Here's how the part is built. I have some questions about the finished solid (model axes, mm). A direction names the side the tool comes from. Round coordinates to 2 decimals unless told otherwise and drop trailing zeros. Loops run counter-clockwise (first coordinate to the right, second up) from the corner with the lowest first, then second, coordinate; pieces in that order, holes last. Notation, with made-up numbers: M 73,84.25 L 78,84.25 A13 cw 78,104.25 Z; hole C 7.5,82 d11. An arc over 180 degrees is marked long. Write each question's results on one line, items separated by ' | '. Start each with the question number.
```python
from build123d import *

# Parameters (mm, degrees)
F0_R     = 0.762
F1_DEPTH = 7.9248
F2_R     = 1.524
F3_DEPTH = 32.005


with BuildPart() as f1:
    # F0 (on Top) → F1 (new body)
    with BuildSketch(Plane.XY):
        Polygon((32.004, 34.163), (32.004, 40.513), (12.319, 40.513), (12.319, 34.29), (5.08, 34.29), (0, 29.21), (0, 0), (6.985, -6.985), (13.589, -6.985), (13.589, -11.303), (16.764, -11.303), (16.764, -6.985), (20.32, -6.985), (20.32, 22.733), align=None)
        with Locations((22.098, 33.909)):
            Circle(F0_R, mode=Mode.SUBTRACT)
    extrude(amount=F1_DEPTH)

    # F2 (on Right) → F3 (cut, through all)
    with BuildSketch(Plane.YZ):
        with Locations((37.3888, 4.064)):
            Circle(F2_R)
        with BuildLine():
            Line((-11.303, 2.54), (-9.3472, 2.54))
            ThreePointArc((-9.3472, 2.54), (-7.8232, 4.064), (-9.3472, 5.588))
            Line((-9.3472, 5.588), (-11.303, 5.588))
            Line((-11.303, 5.588), (-11.303, 2.54))
        make_face()
    extrude(amount=F3_DEPTH, mode=Mode.SUBTRACT)


solid = f1.part
```
1. I need wall thicknesses on line 1 along X through (y, z) = (15.5, 3.75); line 2 along X through (y, z) = (-8, 5); line 3 along Y through (x, z) = (12.5, 6.75) (3 decimals). Which ranges of each line are inside material? Lowest first, please.
2. Which directions (+Z, -Z, +X, -X, +Y, -Y) give clear straight access to the entire face, cutting with the end or side of a thin tool? Please do faces 4 (the face through (15, -10, 5.588)), 5 (the face through (13.589, -8, 3)), 6 (the face through (12.319, 39, 3)).
3. I want a section at B-B on x = 22. List the corners of the cut face in (y, z) for me, plus the area to 3 significant figures.
4. For pin 1 (4 mm diameter, centred on x = 19, z = 4, fed in from -Y) (3 decimals); pin 2 (1.2 mm diameter, centred on x = 22.098, y = 33.909, fed in from -Z); pin 3 (3 mm diameter, centred on x = 18, z = 4, fed in from -Y); pin 4 (4 mm diameter, centred on x = 7, z = 4.5, fed in from +Y), each with a flat end and sliding along its axis, tell me the tip position at first contact or that it passes through.
5. I want a section at D-D on y = 22. List the corners of the cut face in (x, z) for me.
6. If we mould it in two halves opening along Z, with no side actions, what happens to faces 1 (the face through (22.024, 35.866, 4.131)), 2 (the face through (10, -6.985, 4)), 3 (the face through (12, 21, 0))? For each: released by +Z, released by -Z, zero draft, split by the parting line, or undercut.
7. I want a section at C-C on z = 0.5. List the corners of the cut face in (x, y) for me (3 decimals).
8. I want a section at A-A on z = 3.25. List the corners of the cut face in (x, y) for me (3 decimals), plus the area to 3 significant figures.
Outcome:
1) line 1: 0 to 20.32 | line 2: 13.59 to 16.76 | line 3: -6.985 to 40.513
2) face 4: +X, -X, -Y | face 5: +Z, -Z, -X, -Y | face 6: +Z, -Z, -X, +Y
3) outline: M 24.38,0 L 33.15,0 L 33.15,7.92 L 24.38,7.92 Z; M 34.66,0 L 40.51,0 L 40.51,7.92 L 34.66,7.92 Z; hole C 37.39,4.06 d3.05 | area: 109 mm2
4) pin 1: y = -6.985 | pin 2: through | pin 3: y = -8.13 | pin 4: y = 34.29
5) outline: M 0,0 L 20.32,0 L 20.32,7.92 L 0,7.92 Z
6) face 1: undercut | face 2: zero draft | face 3: released by -Z
7) outline: M 0,0 L 6.985,-6.985 L 13.589,-6.985 L 13.589,-11.303 L 16.764,-11.303 L 16.764,-6.985 L 20.32,-6.985 L 20.32,22.733 L 32.004,34.163 L 32.004,40.513 L 12.319,40.513 L 12.319,34.29 L 5.08,34.29 L 0,29.21 Z; hole C 22.098,33.909 d1.524
8) outline: M 0,0 L 6.985,-6.985 L 13.589,-6.985 L 13.589,-8.059 L 16.764,-8.059 L 16.764,-6.985 L 20.32,-6.985 L 20.32,22.733 L 32.004,34.163 L 32.004,36.1 L 12.319,36.1 L 12.319,34.29 L 5.08,34.29 L 0,29.21 Z; M 12.319,38.677 L 32.004,38.677 L 32.004,40.513 L 12.319,40.513 Z; hole C 22.098,33.909 d1.524 | area: 943 mm2
